Input: dimensioned drawing with shaded views. Units: mm. Origin: part minimum x, y, z. A direction names the side the tool comes from. Coordinates: 2 decimals unless noted, no trailing zeros. Order: outer loops, then holes, each group sorted by start corner. A loop starts at its lowest first (then second) coordinate and runs counter-clockwise, first axis right, second up. Notation, with made-up numbers: (84, -18.5) -> (103, -18.5) arc R7 cw to (103, -11.5) -> close; hole circle Ø7 at (-17.75, 18.25). An arc over 180 degrees is marked (long way). Put each result on its own line as item: value.
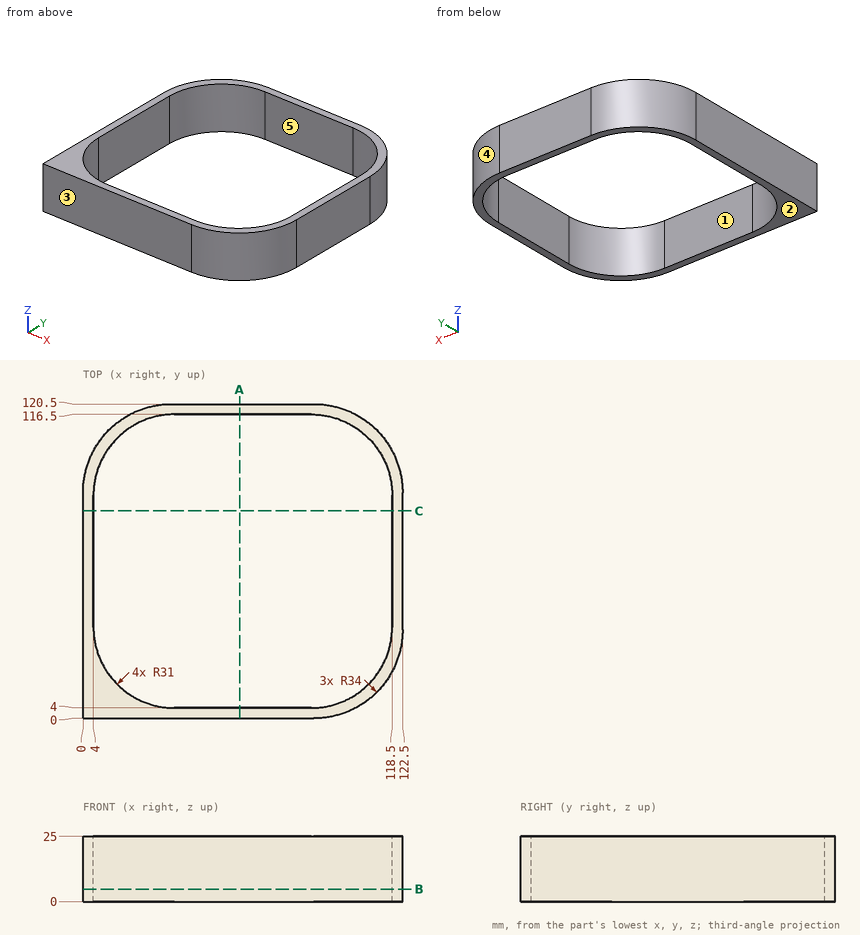
1. Pull-direction query (Y, two-part tool) for the marked faces 1, 2 and 3; classes: pulls with the +Y half, pulls with the -Y half, needs draft (parallel to the pull), parting line crosses it, or undercut.
Numbers:
face 1: undercut
face 2: needs draft
face 3: pulls with the -Y half
2. First-contact query: pin 1 (12 mm diameter, centred on x = 59.5, y = 106.5, fed in from -Z) (3 decimals); pin 2 (6 mm diameter, centred on x = 21, z = 14.5, fed in from +Y); pin 3 (8 mm diameter, centred on x = 104, z = 18.5, fed in from -Y). Flat tips, straight axial feed; report the tip coordinate or a pass-through.
Numbers:
pin 1: passes through
pin 2: stops at y = 119
pin 3: stops at y = 2
3. Set-up query: the marked faces 4 and 5. Return all of +Z, -Z, +X, -X, +Y, -Y with unobstructed straight access to the full face (end or side cutting, diameter ignored); none if empty.
Numbers:
face 4: +Z, -Z, +X, +Y
face 5: +Z, -Z
4. Cut plane B-B on z = 4.75. Output: boundary loops of the cut face in (x, y), plus the area to 3 significant figures.
Numbers:
outline: (0, 0) -> (88.5, 0) arc R34 ccw to (122.5, 34) -> (122.5, 86.5) arc R34 ccw to (88.5, 120.5) -> (34, 120.5) arc R34 ccw to (0, 86.5) -> close; hole (4, 35) arc R31 ccw to (35, 4) -> (87.5, 4) arc R31 ccw to (118.5, 35) -> (118.5, 85.5) arc R31 ccw to (87.5, 116.5) -> (35, 116.5) arc R31 ccw to (4, 85.5) -> close
area: 1,960 mm2
5. Ray query, line 1 along Y through (x, z) = (49.5, 6.5); line 2 along X through (y, z) = (34.5, 8.25); line 3 along Y through (x, z) = (94.5, 11). Return the intervals inside material, ascending.
Numbers:
line 1: y = 0 to 4, 116.5 to 120.5
line 2: x = 0 to 4, 118.5 to 122.5
line 3: y = 0.53 to 4.8, 115.7 to 119.97
6. Cut plane A-A on x = 60. Output: boundary loops of the cut face in (y, z).
Numbers:
outline: (0, 0) -> (4, 0) -> (4, 25) -> (0, 25) -> close; (116.5, 0) -> (120.5, 0) -> (120.5, 25) -> (116.5, 25) -> close
7. Cut plane C-C on y = 79.5. Output: boundary loops of the cut face in (x, z), plus the area to 3 significant figures.
Numbers:
outline: (0, 0) -> (4, 0) -> (4, 25) -> (0, 25) -> close; (118.5, 0) -> (122.5, 0) -> (122.5, 25) -> (118.5, 25) -> close
area: 200 mm2
